Input: part model. Units: mm. Frame: model coordinates. Face numbers are marked on the shaded views. Give positions to 0.01 mm unless a question says otherwise; leave off trailing zeros. Write each loop counter-clockwise with the first axis right and the second up, starting at its lowest first coordinate (ties: lowest second). Pieces come first, ordered by that corner, then holes. Notation, with made-up numbers: (11, 10) - (19, 10) arc R5 cw to (19, 16) - close; hole circle Ø10 at (18.25, 25.25). An arc over 180 degrees is marked (long way). Use a Markdown table: item, result. Add a question column.
1. Section query A-A, the plane z = 0. Return loops of the section in (x, y).
2. Pin query (flat end, axial travel): pin 1 (2 mm diameter, centred on x = -9, y = 17.5, fed in from +Z); pin 2 (2 mm diameter, centred on y = 17.5, z = -23, fed in from +X); pin 3 (6 mm diameter, centred on y = 9, z = -1.5, fed in from -X). Return the tip coordinate at first contact, or that it passes through.
3. Section query C-C, the plane y = 11. Return loops of the section in (x, z), plus the area to 3 significant figures.
4. Material intervals for probe 1 along X at (y, z) = (1.3, 0); probe 2 along X at (y, z) = (21.25, 0), sorted ascending.
5. Section query B-B, the plane x = 0. Return loops of the section in (y, z).
6. Mould query, pull axis Z, two halves, no side actions, for the marked faces 1, 2 and 3. Classes: released by +Z, released by -Z, zero draft, split by the parting line, or undercut.
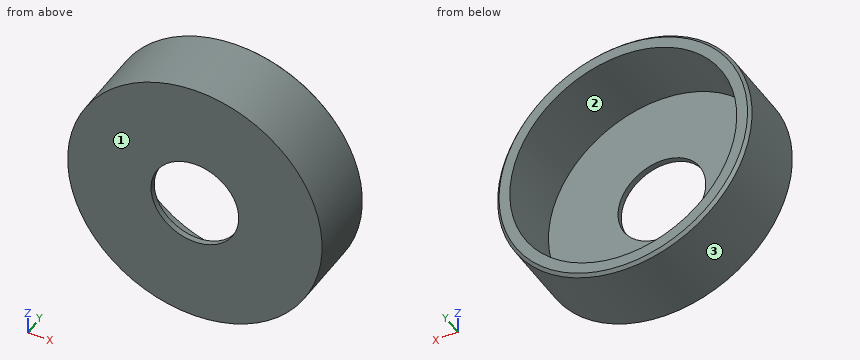
```python
from build123d import *

# Parameters (mm, degrees)
SKETCH_1_R          = 43.5
EXTRUDE_1_DEPTH     = 26
SKETCH_2_R          = 38.8
CUT_EXTRUDE_1_DEPTH = 24
SKETCH_3_R          = 15
CUT_EXTRUDE_2_DEPTH = 67.034082109
CHAMFER_1_SIZE      = 1


with BuildPart() as part:
    # 草图1 → 凸台-拉伸1 (new body)
    with BuildSketch(Plane(origin=(0, 0, 0), x_dir=(1, 0, 0), z_dir=(0, 1, 0))):
        with Locations(Location((0, 0, 0), (0, 0, 90))):
            Circle(SKETCH_1_R)
    extrude(amount=EXTRUDE_1_DEPTH)

    # 草图2 → 切除-拉伸1 (cut)
    with BuildSketch(Plane(origin=(0, 26, 0), x_dir=(1, 0, 0), z_dir=(0, 1, 0))):
        with Locations(Location((0, 0, 0), (0, 0, 270))):
            Circle(SKETCH_2_R)
    extrude(amount=-CUT_EXTRUDE_1_DEPTH, mode=Mode.SUBTRACT)

    # 草图3 → 切除-拉伸2 (cut, through all)
    with BuildSketch(Plane(origin=(0, 2, 0), x_dir=(1, 0, 0), z_dir=(0, 1, 0))):
        with Locations(Location((0, 0, 0), (0, 0, 270))):
            Circle(SKETCH_3_R)
    extrude(amount=-CUT_EXTRUDE_2_DEPTH, mode=Mode.SUBTRACT)

    # 倒角1
    chamfer_1_edges = [part.edges().sort_by_distance(p)[0] for p in [
        (0, 26, 43.5),
    ]]
    chamfer(chamfer_1_edges, length=CHAMFER_1_SIZE)


solid = part.part
```
Result sheet:
| question | item | result |
|---|---|---|
| 1 | outline | (-43.5, 0) - (-15, 0) - (-15, 2) - (-38.8, 2) - (-38.8, 26) - (-42.5, 26) - (-43.5, 25) - close; (15, 0) - (43.5, 0) - (43.5, 25) - (42.5, 26) - (38.8, 26) - (38.8, 2) - (15, 2) - close |
| 2 | pin 1 | stops at z = 42.76 |
| 2 | pin 2 | stops at x = 37.53 |
| 2 | pin 3 | stops at x = -43.5 |
| 3 | outline | circle Ø87 at (0, 0); hole circle Ø77.6 at (0, 0) |
| 3 | area | 1,220 mm² |
| 4 | probe 1 | x = -43.5 to -15, 15 to 43.5 |
| 4 | probe 2 | x = -43.5 to -38.8, 38.8 to 43.5 |
| 5 | outline | (0, -43.5) - (25, -43.5) - (26, -42.5) - (26, -38.8) - (2, -38.8) - (2, -15) - (0, -15) - close; (0, 15) - (2, 15) - (2, 38.8) - (26, 38.8) - (26, 42.5) - (25, 43.5) - (0, 43.5) - close |
| 6 | face 1 | zero draft |
| 6 | face 2 | undercut |
| 6 | face 3 | split by the parting line |
